```python
from build123d import *

# Parameters (mm, degrees)
CROQUIS1_W              = 62
CROQUIS1_H              = 25
SALIENTE_EXTRUIR1_DEPTH = 4
CROQUIS2_W              = 1
CROQUIS2_H              = 15.1
CROQUIS2_H_2            = 13.1
CROQUIS2_W_2            = 0.8
CORTAR_EXTRUIR1_DEPTH   = 2
SALIENTE_EXTRUIR7_START = 2
SALIENTE_EXTRUIR7_DEPTH = 2
CROQUIS6_W              = 6.721970081
CROQUIS6_H              = 7.48208129
SALIENTE_EXTRUIR8_DEPTH = 2
CROQUIS7_W              = 9.9
CROQUIS7_H              = 25
CORTAR_EXTRUIR2_DEPTH   = 2


with BuildPart() as part:
    # Croquis1 → Saliente-Extruir1 (new body)
    with BuildSketch(Plane.XY):
        with Locations((-23.290947876, 17.916666667)):
            Rectangle(CROQUIS1_W, CROQUIS1_H)
    extrude(amount=SALIENTE_EXTRUIR1_DEPTH)

    # Croquis2 → Cortar-Extruir1 (cut)
    # profile 1 of 6: a face of its own
    with BuildSketch(Plane.XY.offset(4)):
        Polygon((5.709052124, 25.616666667), (-44.390947876, 25.616666667), (-44.390947876, 27.616666667), (5.709052124, 27.616666667), (5.709052124, 28.416666667), (-44.390947876, 28.416666667), (-44.390947876, 30.416666667), (-54.290947876, 30.416666667), (-54.290947876, 5.416666667), (-44.390947876, 5.416666667), (-44.390947876, 24.616666667), (5.709052124, 24.616666667), align=None)
    # profile 2 of 6: a face of its own
    with BuildSketch(Plane.XY.offset(4)):
        Polygon((7.209052124, 23.616666667), (-8.669899716, 23.616666667), (-8.669899716, 22.207688927), (-8.669899716, 5.416666667), (7.209052124, 5.416666667), align=None)
        with BuildLine():
            Line((6.152295829, 22.616666667), (-7.669899716, 16.428416464))
            Line((-7.669899716, 16.428416464), (-7.669899716, 9.374881416))
            Line((-7.669899716, 9.374881416), (-5.566552681, 7.979930525))
            ThreePointArc((-5.566552681, 7.979930525), (2.861635527, 13.241627263), (6.152295829, 22.616666667))
        make_face(mode=Mode.SUBTRACT)
        Polygon((-7.669899716, 22.616666667), (3.696371878, 22.616666667), (-7.669899716, 17.52794308), align=None, mode=Mode.SUBTRACT)
    # profile 3 of 6: a face of its own
    with BuildSketch(Plane.XY.offset(4)):
        with Locations((-41.790947876, 12.966666667)):
            Rectangle(CROQUIS2_W, CROQUIS2_H)
    # profile 4 of 6: a face of its own
    with BuildSketch(Plane.XY.offset(4)):
        with Locations((-38.790947876, 11.966666667)):
            Rectangle(CROQUIS2_W, CROQUIS2_H_2)
    # profile 5 of 6: a face of its own
    with BuildSketch(Plane.XY.offset(4)):
        with Locations((-35.890947876, 12.966666667)):
            Rectangle(CROQUIS2_W_2, CROQUIS2_H)
    # profile 6 of 6: a face of its own
    with BuildSketch(Plane.XY.offset(4)):
        with Locations((-33.090947876, 11.966666667)):
            Rectangle(CROQUIS2_W_2, CROQUIS2_H_2)
    extrude(amount=-CORTAR_EXTRUIR1_DEPTH, mode=Mode.SUBTRACT)

    # Croquis4 → Saliente-Extruir7 (add)
    with BuildSketch(Plane.XY.offset(4).offset(SALIENTE_EXTRUIR7_START)):
        with BuildLine():
            Line((-5.566552681, 7.979930525), (-7.669899716, 9.374881416))
            Line((-7.669899716, 9.374881416), (-7.669899716, 16.428416464))
            Line((-7.669899716, 16.428416464), (6.152295829, 22.616666667))
            ThreePointArc((6.152295829, 22.616666667), (2.861635527, 13.241627263), (-5.566552681, 7.979930525))
        make_face()
    extrude(amount=-SALIENTE_EXTRUIR7_DEPTH)

    # Croquis6 → Saliente-Extruir8 (add)
    with BuildSketch(Plane.XY.offset(4)):
        with Locations((-6.543986658, 20.329349066)):
            Rectangle(CROQUIS6_W, CROQUIS6_H)
    extrude(amount=SALIENTE_EXTRUIR8_DEPTH)

    # Croquis7 → Cortar-Extruir2 (cut)
    with BuildSketch(Plane.XY.offset(2)):
        with Locations((-49.340947876, 17.916666667)):
            Rectangle(CROQUIS7_W, CROQUIS7_H)
    extrude(amount=-CORTAR_EXTRUIR2_DEPTH, mode=Mode.SUBTRACT)


solid = part.part
```
Input: part model. Units: mm. Frame: model coordinates. A direction names the side the tool comes from. Give positions to 0.01 mm unless a question says otherwise; leave off trailing zeros. Order: outer loops, then holes, each group sorted by start corner. A loop starts at its lowest first (then second) coordinate and runs counter-clockwise, first axis right, second up.
1. Section A-A on z = 4.5. Return the cut outline in (x, y), and give its area (3 significant figures).
Derived:
outline: (-9.9, 16.59) - (-7.31, 16.59) - (-7.67, 16.43) - (-7.67, 9.37) - (-5.57, 7.98) arc R15 ccw to (6.15, 22.62) - (-3.18, 18.44) - (-3.18, 24.07) - (-9.9, 24.07) - close
area: 161 mm2
2. Reachability of faces 1 (the flat face through (-8.67, 15, 3)), 2 (the flat face through (5.709, 25, 3)), 3 (the flat face through (-9.905, 20, 5)), 4 (the flat face through (-39.291, 12, 3)) from +Z, -Z, +X, -X, +Y, -Y: full face, straight path, thin tool, end or side. Return the list, or none.
Derived:
face 1: -Y
face 2: +Z, -X
face 3: +Z, -X, +Y, -Y
face 4: +Z, -Y
3. Section D-D on x = 3. Return the cut outline in (y, z), and give its area (3 significant figures).
Derived:
outline: (5.42, 0) - (30.42, 0) - (30.42, 4) - (28.42, 4) - (28.42, 2) - (27.62, 2) - (27.62, 4) - (25.62, 4) - (25.62, 2) - (24.62, 2) - (24.62, 4) - (23.62, 4) - (23.62, 2) - (22.62, 2) - (22.62, 4) - (22.3, 4) - (22.3, 2) - (21.21, 2) - (21.21, 6) - (13.42, 6) - (13.42, 2) - (5.42, 2) - close
area: 91.8 mm2
4. Pin query (flat end, axial travel): pin 1 (0.9 mm diameter, centred on x = -19.5, y = 28, fed in from +Z). Return the tip coordinate at first contact, or that it passes through.
Derived:
pin 1: stops at z = 4
5. Section B-B on x = -4. Return the cut outline in (y, z), and give its area (3 significant figures).
Derived:
outline: (5.42, 0) - (30.42, 0) - (30.42, 4) - (28.42, 4) - (28.42, 2) - (27.62, 2) - (27.62, 4) - (25.62, 4) - (25.62, 2) - (24.62, 2) - (24.62, 4) - (24.07, 4) - (24.07, 6) - (8.42, 6) - (8.42, 2) - (5.42, 2) - close; hole (18.07, 2) - (19.17, 2) - (19.17, 4) - (18.07, 4) - close; hole (22.62, 2) - (23.62, 2) - (23.62, 4) - (22.62, 4) - close
area: 117 mm2
6. Material intervals for L1, parallel to Y at x = -37.5, z = 2.2; L2, parallel to Y at x = 4.5, z = 3.5; L3, parallel to X at y = 22.5, z = 2.85, sorted ascending.
Derived:
L1: y = 5.42 to 24.62, 25.62 to 27.62, 28.42 to 30.42
L2: y = 15.77 to 21.88, 23.62 to 24.62, 25.62 to 27.62, 28.42 to 30.42
L3: x = -44.39 to -8.67, -7.67 to 3.44, 5.89 to 6.15, 7.21 to 7.71
7. Section C-C on x = -12.5. Return the cut outline in (y, z), and give its area (3 significant figures).
Derived:
outline: (5.42, 0) - (30.42, 0) - (30.42, 4) - (28.42, 4) - (28.42, 2) - (27.62, 2) - (27.62, 4) - (25.62, 4) - (25.62, 2) - (24.62, 2) - (24.62, 4) - (5.42, 4) - close
area: 96.4 mm2
8. Mould query, pull axis Z, two halves, no side actions, for faces 5 (the flat face through (-1, 21, 4)), 6 (the flat face through (-8, 20, 4)), 7 (the flat face through (-42.291, 13, 3)), 8 (the flat face through (-7.67, 20, 3)). Classes: released by +Z, released by -Z, zero draft, split by the parting line, or undercut.
Derived:
face 5: released by +Z
face 6: undercut
face 7: zero draft
face 8: undercut
